```python
from build123d import *

# Parameters (mm, degrees)
F0_W     = 85.09
F0_H     = 139.7
F1_DEPTH = 6.35
F2_R     = 1.905
F3_DEPTH = 6.351
F4_R     = 2.286
F5_DEPTH = 6.351


with BuildPart() as f1:
    # F0 (on Top) → F1 (new body)
    with BuildSketch(Plane.XY):
        Rectangle(F0_W, F0_H)
    extrude(amount=F1_DEPTH)

    # F2 (on Top) → F3 (cut, through all)
    with BuildSketch(Plane.XY):
        with Locations((-32.22625, -58.208333)):
            Circle(F2_R)
        with Locations((-32.22625, -34.916533)):
            Circle(F2_R)
        with Locations((-32.22625, -11.624733)):
            Circle(F2_R)
        with Locations((-32.22625, 11.667067)):
            Circle(F2_R)
        with Locations((-32.22625, 34.958867)):
            Circle(F2_R)
        with Locations((-32.22625, 58.250667)):
            Circle(F2_R)
        with Locations((-11.60145, -58.208333)):
            Circle(F2_R)
        with Locations((-11.60145, -34.916533)):
            Circle(F2_R)
        with Locations((-11.60145, -11.624733)):
            Circle(F2_R)
        with Locations((-11.60145, 11.667067)):
            Circle(F2_R)
        with Locations((-11.60145, 34.958867)):
            Circle(F2_R)
        with Locations((-11.60145, 58.250667)):
            Circle(F2_R)
        with Locations((9.02335, -58.208333)):
            Circle(F2_R)
        with Locations((9.02335, -34.916533)):
            Circle(F2_R)
        with Locations((9.02335, -11.624733)):
            Circle(F2_R)
        with Locations((9.02335, 11.667067)):
            Circle(F2_R)
        with Locations((9.02335, 34.958867)):
            Circle(F2_R)
        with Locations((9.02335, 58.250667)):
            Circle(F2_R)
        with Locations((29.64815, -58.208333)):
            Circle(F2_R)
        with Locations((29.64815, -34.916533)):
            Circle(F2_R)
        with Locations((29.64815, -11.624733)):
            Circle(F2_R)
        with Locations((29.64815, 11.667067)):
            Circle(F2_R)
        with Locations((29.64815, 34.958867)):
            Circle(F2_R)
        with Locations((29.64815, 58.250667)):
            Circle(F2_R)
    extrude(amount=F3_DEPTH, mode=Mode.SUBTRACT)

    # F4 (on Top) → F5 (cut, through all)
    with BuildSketch(Plane.XY):
        with Locations((-32.22625, -58.208333)):
            Circle(F4_R)
        with Locations((-32.22625, -34.916533)):
            Circle(F4_R)
        with Locations((-32.22625, -11.624733)):
            Circle(F4_R)
        with Locations((-32.22625, 11.667067)):
            Circle(F4_R)
        with Locations((-32.22625, 34.958867)):
            Circle(F4_R)
        with Locations((-32.22625, 58.250667)):
            Circle(F4_R)
    extrude(amount=F5_DEPTH, mode=Mode.SUBTRACT)


solid = f1.part
```
CAD build for the part. Positions are in the model's coordinates, mm. Round coordinates to 2 decimals unless told otherwise and drop trailing zeros. Return JSON: item names as keys, results as strings. Group by question number.
Item 1: Band-saw the part on A-A on z = 3. State how many separate pieces and enclosed holes the cut face has, plus the area to 3 significant figures.
Item 2: Probe probe 1 along X at (y, z) = (34.5, 1) (3 decimals); probe 2 along X at (y, z) = (-57.5, 2.5) (3 decimals). List the from-to ranges inside material, lowest first.
Item 3: Mould opens along Y. For faces 1 (the face through (-1, 1, 6.35)), 2 (the face through (7.62, 36.25, 3.13)) say: +Y half, -Y half, draft (parallel to the pull), parting line (faces both ways), or undercut.
Resolved:
{
 "1": {"separate pieces": "1", "enclosed holes": "24", "area": "11,600 mm²"},
 "2": {"probe 1": "x = -42.545 to -34.466, -29.987 to -13.45, -9.753 to 7.174, 10.872 to 27.799, 31.497 to 42.545", "probe 2": "x = -42.545 to -34.4, -30.053 to -13.37, -9.833 to 7.255, 10.792 to 27.88, 31.417 to 42.545"},
 "3": {"face 1": "draft", "face 2": "undercut"}
}
